Input: part model. Units: mm. Frame: model coordinates. Face numbers are marked on the shaded views. Round coordinates to 2 decimals unless told otherwise and drop trailing zeros. Write each loop counter-clockwise with the first axis right and the second up, starting at its lowest first coordinate (ties: lowest second). Pieces come first, ordered by that corner, then holes. Notation, with made-up numbers: (40, 4) -> (70, 4) arc R23 cw to (70, 30) -> close; hole circle Ø2 at (41, 48). An arc over 180 degrees is marked (long way). Write item = value, one per line.
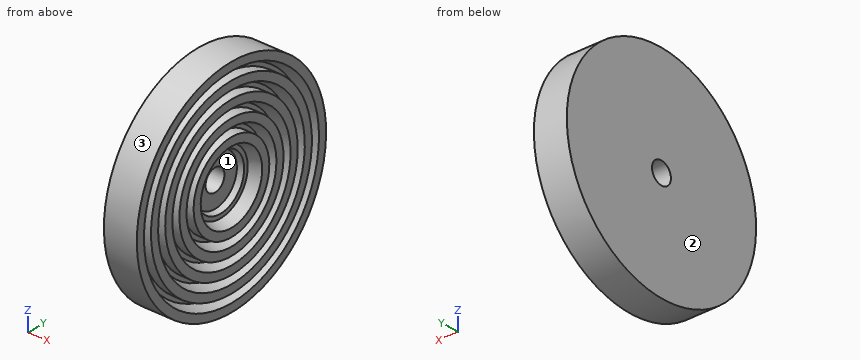
```python
from build123d import *


with BuildPart() as part:
    # Schizzo3 → Rivoluzione1 (revolve)
    with BuildSketch(Plane.XY, mode=Mode.PRIVATE) as rivoluzione1_sk:
        Polygon((0, 0), (0, 18), (6, 18), (6, 16.5), (4, 15.75), (4, 15), (6, 15), (6, 13.5), (4, 12.75), (4, 12), (6, 12), (6, 10.5), (4, 9.75), (4, 9), (6, 9), (6, 7.5), (4, 6.75), (4, 6), (6, 6), (6, 4.5), (4, 3.75), (4, 3), (3, 2.625), (3, 0), align=None)
    revolve(rivoluzione1_sk.sketch.rotate(Axis((-0.664443358, -2, 0), (1, 0, 0)), 90), axis=Axis((-0.664443358, -2, 0), (1, 0, 0)))


solid = part.part
```
1) First-contact query: P1, Ø3.5, axis at y = -1, z = 1, coming from the +X side. Flat tip, straight axial feed; report the tip coordinate or a pass-through.
Solutions:
P1 = 3
2) Draft query along Z for the marked faces 1, 2 and 3. Return one class per face: +Z half, -Z half, draft (parallel to the pull), parting line (faces both ways), or undercut.
Solutions:
face_1 = undercut
face_2 = draft
face_3 = parting line
3) Cut plane A-A (x = 2.4). Return the cut outline in (y, z).
Solutions:
outline = circle Ø40 at (-2, 0); hole circle Ø4 at (-2, 0)
4) Line query: L1, parallel to Z at x = 4.65, y = 11; L2, parallel to Y at x = 0.65, z = 0; L3, parallel to X at y = -7, z = 10. Output: solid intervals per line, ascending. Write a range as from..to.
Solutions:
L1 = -15.2..-12.44, -10.95..-7.47, -5.2..5.2, 7.47..10.95, 12.44..15.2
L2 = -22..-4, 0..18
L3 = 0..4
